Geometry: final body of the model. Coordinates: model frame, mm. Give positions to 0.01 mm unless a question says otherwise; leave off trailing zeros. Order: outer loops, then holes, each group sorted by start corner. A loop starts at its lowest first (then second) coordinate and runs counter-clockwise, first axis right, second up. Notation, with made-up numbers: M 71,57.25 L 81,57.25 A19 cw 81,61.25 Z; hole C -17,38 d10. An arc over 180 degrees is marked long. One line per item, written item: value. Start each with the question number.
```python
from build123d import *

# Parameters (mm, degrees)
EXTRUDE1_DEPTH          = 7.9375
EXTRUDE1_DEPTH_BACK     = 7.9375
SKETCH1_R               = 2.413
SKETCH8_OUTSIDE_W       = 76.264
SKETCH8_OUTSIDE_H       = 77.492
SKETCH8_OUTSIDE_R       = 3.96875
EXTRUDE4_DEPTH          = 17.993172266
EXTRUDE4_DRAFT          = -60
MIRROR1_COPY_1_SKETCH_W = 76.264
MIRROR1_COPY_1_SKETCH_H = 77.492
MIRROR1_COPY_1_SKETCH_R = 3.96875
MIRROR1_COPY_1_DEPTH    = 17.993172266
MIRROR1_COPY_1_DRAFT    = -60


with BuildPart() as part:
    # Sketch1 → Extrude1 (new, two sides: drawn at the far end of the back side and taken through both)
    with BuildSketch(Plane.XY.offset(-EXTRUDE1_DEPTH_BACK)):
        Polygon((0, 4.582717762), (-3.96875, 2.291358881), (-3.96875, -2.291358881), (0, -4.582717762), (3.96875, -2.291358881), (3.96875, 2.291358881), align=None)
        Circle(SKETCH1_R, mode=Mode.SUBTRACT)
    extrude(amount=EXTRUDE1_DEPTH + EXTRUDE1_DEPTH_BACK)

    # Extrude3 cone 1 section (through the dimple's axis) → Extrude3 (revolve, cut)
    with BuildSketch(Plane(origin=(0, 0, -7.9375), x_dir=(0, 1, 0), z_dir=(1, 0, 0))):
        Polygon((0, 0), (2.4638, 0), (0, 2.642102028), align=None)
    extrude3 = revolve(axis=Axis((0, 0, -7.9375), (0, 0, 1)), mode=Mode.SUBTRACT)


with BuildPart() as extrude4_tool:
    # Sketch8 outside → Extrude4 (with draft: the straight prism first)
    with BuildSketch(Plane(origin=(0, 0, -7.9375), x_dir=(-1, 0, 0), z_dir=(0, 0, -1))):
        Rectangle(SKETCH8_OUTSIDE_W, SKETCH8_OUTSIDE_H)
        Circle(SKETCH8_OUTSIDE_R, mode=Mode.SUBTRACT)
    extrude(amount=-EXTRUDE4_DEPTH)
    # Extrude4: the draft: its side faces are tilted about the plane it starts from
    extrude4_sides = [extrude4_tool.faces().sort_by_distance(p)[0] for p in [
        (0, -38.746, 1.059086133),
        (-38.132, 0, 1.059086133),
        (0, 38.746, 1.059086133),
        (38.132, 0, 1.059086133),
        (3.96875, 0, 1.059086133),
    ]]
    draft(extrude4_sides, Plane(origin=(0, 0, -7.9375), x_dir=(-1, 0, 0), z_dir=(0, 0, -1)), EXTRUDE4_DRAFT)


with BuildPart() as part_1:
    add(part.part)

    # Extrude4: cut by extrude4_tool
    add(extrude4_tool.part, mode=Mode.SUBTRACT)

    # Mirror1: Extrude3 across plane
    add(extrude3.mirror(Plane.XY), mode=Mode.SUBTRACT)


with BuildPart() as mirror1_copy_1_tool:
    # Mirror1 copy 1 sketch → Mirror1 copy 1 (with draft: the straight prism first)
    with BuildSketch(Plane(origin=(0, 0, 7.9375), x_dir=(-1, 0, 0), z_dir=(0, 0, 1))):
        Rectangle(MIRROR1_COPY_1_SKETCH_W, MIRROR1_COPY_1_SKETCH_H)
        Circle(MIRROR1_COPY_1_SKETCH_R, mode=Mode.SUBTRACT)
    extrude(amount=-MIRROR1_COPY_1_DEPTH)
    # Mirror1 copy 1: the draft: its side faces are tilted about the plane it starts from
    mirror1_copy_1_sides = [mirror1_copy_1_tool.faces().sort_by_distance(p)[0] for p in [
        (0, -38.746, -1.059086133),
        (-38.132, 0, -1.059086133),
        (0, 38.746, -1.059086133),
        (38.132, 0, -1.059086133),
        (3.96875, 0, -1.059086133),
    ]]
    draft(mirror1_copy_1_sides, Plane(origin=(0, 0, 7.9375), x_dir=(-1, 0, 0), z_dir=(0, 0, 1)), MIRROR1_COPY_1_DRAFT)


with BuildPart() as part_2:
    add(part_1.part)

    # Mirror1 copy 1: cut by mirror1_copy_1_tool
    add(mirror1_copy_1_tool.part, mode=Mode.SUBTRACT)


solid = part_2.part
```
Q1. Contact query for flat-ended pins moving along their axis: pin 1 (1.5 mm diameter, centred on x = 1.5, z = 1, fed in from +Y); pin 2 (2 mm diameter, centred on x = 2.5, z = 0.5, fed in from -Y); pin 3 (3 mm diameter, centred on x = 0, y = 1, fed in from -Z); pin 4 (4.5 mm diameter, centred on x = 0, y = 0, fed in from -Z). Output: stop coordinate, or through.
Q2. Ray query, line 1 along X through (y, z) = (0, -3.25); line 2 along Y through (x, z) = (-1.25, 2.25); line 3 along Y through (x, z) = (1, 3.5). Return the intervals inside material, ascending. Write a range as [from, to].
Q3. Mould query, pull axis X, two halves, no side actions, for faces 1 (the face through (3.56, -2.07, 7.85)), 2 (the face through (-1.915, -1.468, -0.11)), 3 (the face through (-3.969, 0, 0)). Classes: +X half, -X half, draft (parallel to the pull), parting line (faces both ways), or undercut.
Q4. Section query A-A on z = 5. Return loops of the section in (x, y).
Results below:
1. pin 1: y = 4.15
1. pin 2: y = -3.72
1. pin 3: z = -7.94
1. pin 4: through
2. line 1: [-3.97, -2.41], [2.41, 3.97]
2. line 2: [-3.86, -2.06], [2.06, 3.86]
2. line 3: [-4.01, -2.2], [2.2, 4.01]
3. face 1: +X half
3. face 2: undercut
3. face 3: -X half
4. outline: M -3.97,-2.29 L 0,-4.58 L 3.97,-2.29 L 3.97,2.29 L 0,4.58 L -3.97,2.29 Z; hole C 0,0 d4.83
